```python
from build123d import *

# Parameters (mm, degrees)
SKETCH1_R           = 3.65
BOSS_EXTRUDE1_DEPTH = 1.975
SKETCH2_OUTSIDE_W   = 11.51
SKETCH2_OUTSIDE_H   = 11.51
SKETCH2_OUTSIDE_R   = 2.9
CUT_EXTRUDE1_DEPTH  = 0.65


with BuildPart() as part:
    # Sketch1 → Boss-Extrude1 (new, symmetric)
    with BuildSketch(Plane.XY):
        Circle(SKETCH1_R)
        with BuildLine():
            ThreePointArc((0.9, -2.224859546), (0, -2.4), (-0.9, -2.224859546))
            Line((-0.9, -2.224859546), (-0.9, -0.9))
            Line((-0.9, -0.9), (-2.224859546, -0.9))
            ThreePointArc((-2.224859546, -0.9), (-2.4, 0), (-2.224859546, 0.9))
            Line((-2.224859546, 0.9), (-0.9, 0.9))
            Line((-0.9, 0.9), (-0.9, 2.224859546))
            ThreePointArc((-0.9, 2.224859546), (0, 2.4), (0.9, 2.224859546))
            Line((0.9, 2.224859546), (0.9, 0.9))
            Line((0.9, 0.9), (2.224859546, 0.9))
            ThreePointArc((2.224859546, 0.9), (2.4, 0), (2.224859546, -0.9))
            Line((2.224859546, -0.9), (0.9, -0.9))
            Line((0.9, -0.9), (0.9, -2.224859546))
        make_face(mode=Mode.SUBTRACT)
    extrude(amount=BOSS_EXTRUDE1_DEPTH, both=True)

    # Sketch2 outside → Cut-Extrude1 (cut, symmetric)
    with BuildSketch(Plane.XY):
        Rectangle(SKETCH2_OUTSIDE_W, SKETCH2_OUTSIDE_H)
        Circle(SKETCH2_OUTSIDE_R, mode=Mode.SUBTRACT)
    extrude(amount=CUT_EXTRUDE1_DEPTH, both=True, mode=Mode.SUBTRACT)


solid = part.part
```
CAD build for the part. Positions are in the model's coordinates, mm. A direction names the side the tool comes from. Coordinates: 2 decimals unless noted, no trailing zeros. Write each loop counter-clockwise with the first axis right and the second up, starting at its lowest first coordinate (ties: lowest second). Pieces come first, ordered by that corner, then holes. Notation, with made-up numbers: (35.25, 44.25) -> (88.25, 44.25) arc R14 ccw to (88.25, 64.25) -> close; hole circle Ø5 at (-36, 18). An arc over 180 degrees is marked (long way). Use CSV: the item, a comma, the result in double quotes. Start each with the question number.
Item 1: Drop flat-ended pins along their axis: P1, Ø1.5, axis at y = 2.5, z = -1, coming from the -X side; P2, Ø0.7, axis at x = -1.5, z = -1, coming from the +Y side; P3, Ø0.7, axis at y = -1.5, z = -0.5, coming from the +X side. Give the stop position or say it passes through.
Item 2: Two-plate mould, pull along X, no slides. Class faces 1 (the cylindrical face through (-2.9, 0.1, 0)), 2 (the flat face through (1, 3, 0.65)), 3 (the flat face through (-0.9, -2, 0)): +X half, -X half, draft (parallel to the pull), parting line (faces both ways), or undercut.
Item 3: Wall check: probe 1 along Z at (x, y) = (0, 3.25) (3 decimals); probe 2 along X at (y, z) = (-2, 0.25); probe 3 along Y at (x, z) = (-2.75, -1.2). Give the ranges that are in metal, low to high.
Item 4: Band-saw the part on D-D, the plane y = 2.75. Write the cut outline in (x, z) (3 decimals).
Item 5: Tool access for faces 4 (the flat face through (0.9, 2, 0)), 5 (the flat face through (2, -2, -1.975)), 6 (the flat face through (1, 3, -0.65)): list every direction of +Z, -Z, +X, -X, +Y, -Y with a clear straight run to the whole face (end or side of a thin tool).
Item 6: Band-saw the part on B-B, the plane z = -0.55. Write the cut outline in (x, y).
Item 7: Band-saw the part on A-A, the plane y = 0. Write the cut outline in (x, z) (3 decimals), plus the area to 4 significant figures.
Response values:
1,P1,"stops at x = -3.2"
1,P2,"stops at y = 3.46"
1,P3,"stops at x = 3.45"
2,face 1,"parting line"
2,face 2,"draft"
2,face 3,"undercut"
3,probe 1,"z = -1.975 to -0.65, 0.65 to 1.975"
3,probe 2,"x = -2.1 to -0.9, 0.9 to 2.1"
3,probe 3,"y = -2.4 to 2.4"
4,outline,"(-2.4, -1.975) -> (2.4, -1.975) -> (2.4, -0.65) -> (0.921, -0.65) -> (0.921, 0.65) -> (2.4, 0.65) -> (2.4, 1.975) -> (-2.4, 1.975) -> (-2.4, 0.65) -> (-0.921, 0.65) -> (-0.921, -0.65) -> (-2.4, -0.65) -> close"
5,face 4,"+Z, -Z"
5,face 5,"-Z, +X, -X, +Y, -Y"
5,face 6,"none"
6,outline,"circle Ø5.8 at (0, 0); hole (-2.22, -0.9) -> (-0.9, -0.9) -> (-0.9, -2.22) arc R2.4 ccw to (0.9, -2.22) -> (0.9, -0.9) -> (2.22, -0.9) arc R2.4 ccw to (2.22, 0.9) -> (0.9, 0.9) -> (0.9, 2.22) arc R2.4 ccw to (-0.9, 2.22) -> (-0.9, 0.9) -> (-2.22, 0.9) arc R2.4 ccw to start"
7,outline,"(-3.65, -1.975) -> (-2.4, -1.975) -> (-2.4, 1.975) -> (-3.65, 1.975) -> (-3.65, 0.65) -> (-2.9, 0.65) -> (-2.9, -0.65) -> (-3.65, -0.65) -> close; (2.4, -1.975) -> (3.65, -1.975) -> (3.65, -0.65) -> (2.9, -0.65) -> (2.9, 0.65) -> (3.65, 0.65) -> (3.65, 1.975) -> (2.4, 1.975) -> close"
7,area,"7.925 mm2"
